Part print with two shaded views. Sizes in mm from the minimum x, y, z corner. Give positions to 0.01 mm unless a question says otherwise; leave off trailing zeros. Loops run counter-clockwise (first coordinate to the right, second up) from the corner with the lowest first, then second, coordinate; pieces in that order, holes last. Notation, with made-up numbers: M 18.5,87 L 37.5,87 A25 cw 37.5,122 Z; hole C 34,66.5 d5. An arc over 180 degrees is marked long. Answer as a JSON object with one key per item and string values. Group by question number.
1. Slice it at A-A (x = 279.4). List the corners of the cut face in (y, z), then the cut area to 3 significant figures.
2. Mould opens along Y. For the marked faces 1, 2 and 3 say: released by +Y, released by -Y, zero draft, split by the parting line, or undercut.
3. Drill centre lines: line 1 along Y through (x, z) = (279, 177); line 2 along X through (y, z) = (146, 294). Where is each one in solid material? Low to high. Write a range as [from, to].
4. Drop flat-ended pins along their axis: pin 1 Ø2 at (y, z) = (177, 227) entering from -X; pin 2 Ø1.5 at (x, z) = (165, 95.5) entering from +Y; pin 3 Ø6 at (x, z) = (273, 60) entering from +Y. Give the stop position or say it passes through.
5. Slice it at C-C (z = 176.5). List the corners of the cut face in (x, y), then the cut area to 3 significant figures.
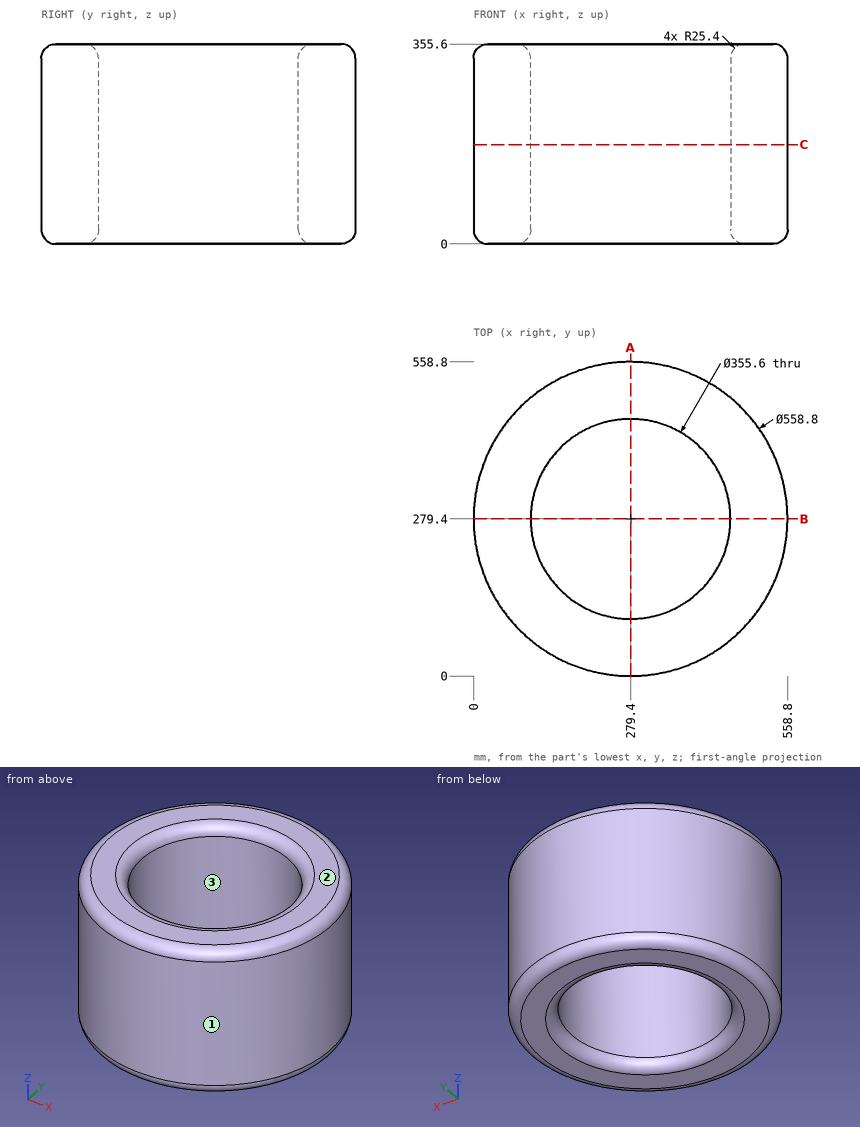
Established:
{
 "1": {"outline": "M 0,25.4 A25.4 ccw 25.4,0 L 76.2,0 A25.4 ccw 101.6,25.4 L 101.6,330.2 A25.4 ccw 76.2,355.6 L 25.4,355.6 A25.4 ccw 0,330.2 Z; M 457.2,25.4 A25.4 ccw 482.6,0 L 533.4,0 A25.4 ccw 558.8,25.4 L 558.8,330.2 A25.4 ccw 533.4,355.6 L 482.6,355.6 A25.4 ccw 457.2,330.2 Z", "area": "71,200 mm^2"},
 "2": {"face 1": "split by the parting line", "face 2": "zero draft", "face 3": "undercut"},
 "3": {"line 1": "y = [0, 101.6], [457.2, 558.8]", "line 2": "x = [33.9, 161.85], [396.95, 524.9]"},
 "4": {"pin 1": "stops at x = 19.05", "pin 2": "stops at y = 534.64", "pin 3": "stops at y = 558.78"},
 "5": {"outline": "C 279.4,279.4 d558.8; hole C 279.4,279.4 d355.6", "area": "146,000 mm^2"}
}
